```python
from build123d import *

# Parameters (mm, degrees)
SKETCH1_R           = 1.35
BOSS_EXTRUDE1_DEPTH = 3


with BuildPart() as part:
    # Sketch1 → Boss-Extrude1 (new body)
    with BuildSketch(Plane(origin=(0, 0, 0), x_dir=(1, 0, 0), z_dir=(0, 1, 0))):
        with BuildLine():
            Line((280, 50), (25, 50))
            ThreePointArc((25, 50), (0.080648745, 27.00647278), (21, 0.322074641))
            ThreePointArc((21, 0.322074641), (150.709603392, -8.943952981), (280, 5))
            ThreePointArc((280, 5), (296.028917332, 15.902478251), (299.356812448, 35))
            ThreePointArc((299.356812448, 35), (292.244245466, 45.811097932), (280, 50))
        make_face()
        with Locations(Location((19.343145751, 30.656854249, 0), (0, 0, 270))):
            Circle(SKETCH1_R, mode=Mode.SUBTRACT)
        with Locations(Location((30.656854249, 30.656854249, 0), (0, 0, 270))):
            Circle(SKETCH1_R, mode=Mode.SUBTRACT)
        with Locations(Location((19.343145751, 19.343145751, 0), (0, 0, 270))):
            Circle(SKETCH1_R, mode=Mode.SUBTRACT)
        with Locations(Location((30.656854249, 19.343145751, 0), (0, 0, 270))):
            Circle(SKETCH1_R, mode=Mode.SUBTRACT)
    extrude(amount=BOSS_EXTRUDE1_DEPTH)


solid = part.part
```
The listing builds one solid part. Answer for the finished solid, in the listing's coordinates (mm). Give positions to 0.01 mm unless a question says otherwise; leave off trailing zeros. Order: outer loops, then holes, each group sorted by start corner. A loop starts at its lowest first (then second) coordinate and runs counter-clockwise, first axis right, second up.
1) Find section A-A on y = 1.2. Write down the section's boundary in (x, z), then the cut area to 3 significant figures.
Reported:
outline: (21, -0.32) arc R25 ccw to (25, -50) - (280, -50) arc R19.99 ccw to (299.36, -35) arc R24.86 ccw to (280, -5) arc R728.47 ccw to start; hole circle Ø2.7 at (19.34, -30.66); hole circle Ø2.7 at (19.34, -19.34); hole circle Ø2.7 at (30.66, -30.66); hole circle Ø2.7 at (30.66, -19.34)
area: 15,700 mm2
2) Consider line 1 along X through (y, z) = (0.9, -31); line 2 along X through (y, z) = (1.05, -37.5); line 3 along Z through (x, y) = (222, 2.7). Determine where each line is inside the solid, lowest interval first.
Reported:
line 1: x = 0.73 to 18.04, 20.65 to 29.35, 31.96 to 299.95
line 2: x = 3.35 to 298.53
line 3: z = -50 to 4.15
3) Given P1, Ø12, axis at x = 223, z = -1, coming from the -Y side; P2, Ø1, axis at y = 2, z = -25.5, coming from the -X side; P3, Ø2, axis at x = 19.34, z = -30.66, coming from the +Y side, each flat-ended and moving along its own axis, determine where each tip first touches the part or whether it passes through.
Reported:
P1: stops at y = 0
P2: stops at x = 0
P3: passes through
4) Find section C-C on z = -46. Write down the section's boundary in (x, y).
Reported:
outline: (11.44, 0) - (292, 0) - (292, 3) - (11.44, 3) - close
5) Find section B-B on x = 83. Write down the section's boundary in (y, z).
Reported:
outline: (0, -50) - (3, -50) - (3, 7.02) - (0, 7.02) - close
